Work out the finished part from the listing and answer in its coordinate system (mm). A direction names the side the tool comes from. Give positions to 0.01 mm unless a question says otherwise; leave off trailing zeros. Loops run counter-clockwise (first coordinate to the right, second up) from the corner with the lowest first, then second, coordinate; pieces in that order, holes last. Notation, with made-up numbers: M 18,38.5 L 67,38.5 A23 ccw 67,50.5 Z; hole C -14.5,62.5 d4. An arc over 180 degrees is marked long. Answer in a Markdown table with one row per item. Add a question column.
Autodesk Inventor part; units mm, degrees
ref_plane "YZ Plane" through (0, 0, 0) normal (1, 0, 0) x (0, 1, 0)
ref_plane "XZ Plane" through (0, 0, 0) normal (0, 1, 0) x (-1, 0, 0)
ref_plane "XY Plane" through (0, 0, 0) normal (0, 0, 1) x (1, 0, 0)
sketch "Block1" plane through (0, 0, 0) normal (0, 0, 1) x (1, 0, 0)
  circle A0 centre (74.029, 24.2723) radius 1
  line L0 (49.279, 30.4723) -> (71.779, 30.4723)
  line L1 (71.779, 30.4723) -> (71.779, 18.0723)
  line L2 (71.779, 18.0723) -> (49.279, 18.0723)
  line L3 (49.279, 18.0723) -> (49.279, 30.4723)
  line L4 (49.279, 30.4723) -> (44.779, 30.4723)
  line L5 (44.779, 30.4723) -> (44.779, 18.0723)
  line L6 (44.779, 18.0723) -> (49.279, 18.0723)
  line L7 (49.279, 18.0723) -> (49.279, 30.4723)
  line L8 (71.779, 30.4723) -> (76.279, 30.4723)
  line L9 (76.279, 30.4723) -> (76.279, 18.0723)
  line L10 (76.279, 18.0723) -> (71.779, 18.0723)
  line L11 (71.779, 18.0723) -> (71.779, 30.4723)
  line L12 (44.779, 24.2723) -> (76.279, 24.2723) construction
  line L13 (47.029, 30.4723) -> (47.029, 18.0723) construction
  circle A1 centre (47.029, 24.2723) radius 1
  line L14 (74.029, 30.4723) -> (74.029, 18.0723) construction
  point P0 (60.979, 24.0984)
  dimension "d7" = 22.5
  dimension "d8" = 12.4
  dimension "d9" = 4.5
  dimension "d10" = 4.5
  dimension "d11" = 2
  dimension "d12" = 2
sketch "Sketch1" plane through (0, 0, 0) normal (0, 0, 1) x (1, 0, 0)
  line L0 (-92.7646, -8.503) -> (-89.7646, -8.503)
  line L1 (-89.7646, -8.503) -> (-89.7646, -11.753)
  line L2 (-89.7646, -11.753) -> (-92.7646, -11.753)
  line L3 (-92.7646, -11.753) -> (-92.7646, -8.503)
  line L4 (-92.7646, -21.6527) -> (-89.7646, -21.6527)
  line L5 (-89.7646, -21.6527) -> (-89.7646, -21.7527)
  line L6 (-89.7646, -21.7527) -> (-92.7646, -21.7527)
  line L7 (-92.7646, -21.7527) -> (-92.7646, -21.6527)
  line L8 (18.2857, 30.9706) -> (51.7857, 30.9706)
  line L9 (51.7857, 30.9706) -> (51.7857, 0.7206)
  line L10 (51.7857, 0.7206) -> (18.2857, 0.7206)
  line L11 (18.2857, 0.7206) -> (18.2857, 30.9706)
  line L12 (18.2857, 22.8456) -> (21.5357, 22.8456)
  line L13 (21.5357, 22.8456) -> (21.5357, 8.8456)
  line L14 (21.5357, 8.8456) -> (18.2857, 8.8456)
  line L15 (18.2857, 8.8456) -> (18.2857, 22.8456)
  line L16 (35.0357, 30.9706) -> (35.0357, 0.7206) construction
  line L17 (51.7857, 22.8456) -> (48.5357, 22.8456)
  line L18 (48.5357, 22.8456) -> (48.5357, 8.8456)
  line L19 (48.5357, 8.8456) -> (51.7857, 8.8456)
  line L20 (51.7857, 8.8456) -> (51.7857, 22.8456)
  line L21 (32.5357, -2.5294) -> (37.5357, -2.5294)
  line L22 (37.5357, -2.5294) -> (37.5357, 0.7206)
  line L23 (37.5357, 0.7206) -> (32.5357, 0.7206)
  line L24 (32.5357, 0.7206) -> (32.5357, -2.5294)
  line L25 (35.0357, 0.7206) -> (35.0357, -2.5294) construction
  line L26 (18.2857, 14.2206) -> (51.7857, 14.2206) construction
  line L27 (32.5357, 30.9706) -> (37.5357, 30.9706)
  line L28 (37.5357, 30.9706) -> (37.5357, 27.7206)
  line L29 (37.5357, 27.7206) -> (32.5357, 27.7206)
  line L30 (32.5357, 27.7206) -> (32.5357, 30.9706)
  line L31 (35.0357, 27.7206) -> (35.0357, 30.9706) construction
  line L32 (18.2857, 0.7206) -> (51.7857, 0.7206)
  line L33 (51.7857, 0.7206) -> (51.7857, -2.5294)
  line L34 (51.7857, -2.5294) -> (18.2857, -2.5294)
  line L35 (18.2857, -2.5294) -> (18.2857, 0.7206)
  line L36 (18.2857, -2.5294) -> (21.5357, -2.5294)
  line L37 (21.5357, -2.5294) -> (21.5357, 0.7206)
  line L38 (21.5357, 0.7206) -> (18.2857, 0.7206)
  line L39 (18.2857, 0.7206) -> (18.2857, -2.5294)
  line L40 (51.7857, -2.5294) -> (48.5357, -2.5294)
  line L41 (48.5357, -2.5294) -> (48.5357, 0.7206)
  line L42 (48.5357, 0.7206) -> (51.7857, 0.7206)
  line L43 (51.7857, 0.7206) -> (51.7857, -2.5294)
  point P0 (0, 0)
  point P1 (35.0357, 27.7206)
  dimension "d0" = 3
  dimension "mat" = 3.25
  dimension "d2" = 3
  dimension "d3" = 0.1
  dimension "d32" = 33.5
  dimension "d34" = 3.25
  dimension "d35" = 14
  dimension "d36" = 8.125
  dimension "d39" = 5
  dimension "d40" = 3.25
  dimension "d45" = 8.125
  dimension "d46" = 3.25
extrude "Extrusion3" add sketch "Sketch1" along normal blind 3.25 contours L8 L30 L29 L28 L9 L17 L18 L19 L10 L11 L14 L13 L12 | L8 L28 L29 L30
extrude "Extrusion6" add sketch "Sketch1" along normal blind 3.25 contours L10 L37 L34 L35 | L10 L24 L34 L37 | L33 L34 L41 L10 | L10 L41 L34 L22
extrude "Extrusion7" cut sketch "Sketch1" along normal blind 3.25 contours L10 L37 L34 L35 | L33 L34 L41 L10
extrude "Extrusion8" cut sketch "Sketch1" along normal blind 3.25 contours L8 L28 L29 L30
equation "\"d34\" = mat"
equation "\"d40\" = mat"
equation "\"d46\" = mat"
equation "\"d37\" = mat"
equation "\"d47\" = mat"
equation "\"d49\" = mat"
equation "\"d51\" = mat"
properties part number "arm-servo"
(1) Consider line 1 along X through (y, z) = (0, 0.85); line 2 along Y through (x, z) = (21, 2.1); line 3 along X through (y, z) = (10, 2.6). Determine where each line is inside the solid, lowest interval first. Write a range as from..to.
(2) Each of these flat-tipped pins is pushed along its axis until it touches: P1, Ø1, axis at y = 15, z = 1, coming from the -X side; P2, Ø1, axis at x = 19.5, z = 1, coming from the -Y side; P3, Ø1, axis at x = 34.5, z = 1, coming from the +Y side. Where does it stop, or does it pass through?
(3) Section B-B, the plane z = 1.9 is taken. Determine the outline of the cut face in (x, y), and give its area (3 significant figures).
(4) Section C-C, the plane x = 33 is taken. Determine the outline of the cut face in (y, z).
(5) Which of the six approach directions +Z, -Z, +X, -X, +Y, -Y give full straight-line access (tool end or side, diameter ignored) to faces 1 (the face through (37.536, 29, 2)), 2 (the face through (35, 0.721, 2)), 3 (the face through (21.536, -1, 2))?
(6) Section A-A, the plane y = 29 is taken. Determine the outline of the cut face in (x, z), and give its area (3 significant figures).
(7) The mould has two halves that part along Y. Classify faces 4 (the face through (32.536, -1, 2)), 5 (the face through (50, 8.846, 2)), 6 (the face through (48.536, 16, 2)), 7 (the face through (50, 0.721, 2)): pulls with the +Y half, pulls with the -Y half, needs draft (parallel to the pull), parting line crosses it, or undercut.
(8) Section D-D, the plane y = 20 is taken. Determine the outline of the cut face in (x, z), and give its area (4 significant figures).
Numbers:
| question | item | result |
|---|---|---|
| 1 | line 1 | x = 21.54..32.54, 37.54..48.54 |
| 1 | line 2 | y = 0.72..8.85, 22.85..30.97 |
| 1 | line 3 | x = 21.54..48.54 |
| 2 | P1 | stops at x = 21.54 |
| 2 | P2 | stops at y = 0.72 |
| 2 | P3 | stops at y = 27.72 |
| 3 | outline | M 18.29,0.72 L 21.54,0.72 L 21.54,-2.53 L 32.54,-2.53 L 32.54,0.72 L 37.54,0.72 L 37.54,-2.53 L 48.54,-2.53 L 48.54,0.72 L 51.79,0.72 L 51.79,8.85 L 48.54,8.85 L 48.54,22.85 L 51.79,22.85 L 51.79,30.97 L 37.54,30.97 L 37.54,27.72 L 32.54,27.72 L 32.54,30.97 L 18.29,30.97 L 18.29,22.85 L 21.54,22.85 L 21.54,8.85 L 18.29,8.85 Z |
| 3 | area | 978 mm² |
| 4 | outline | M 0.72,0 L 27.72,0 L 27.72,3.25 L 0.72,3.25 Z |
| 5 | face 1 | +Z, -Z, +Y |
| 5 | face 2 | +Z, -Z, -Y |
| 5 | face 3 | +Z, -Z, -X, -Y |
| 6 | outline | M 18.29,0 L 32.54,0 L 32.54,3.25 L 18.29,3.25 Z; M 37.54,0 L 51.79,0 L 51.79,3.25 L 37.54,3.25 Z |
| 6 | area | 92.6 mm² |
| 7 | face 4 | needs draft |
| 7 | face 5 | undercut |
| 7 | face 6 | undercut |
| 7 | face 7 | pulls with the -Y half |
| 8 | outline | M 21.54,0 L 48.54,0 L 48.54,3.25 L 21.54,3.25 Z |
| 8 | area | 87.75 mm² |
